For this review, use the dimensioned drawing (mm, ordinates from the lowest corner) and the shaded views. A direction names the side the tool comes from. Coordinates: 2 decimals unless noted, no trailing zeros. Order: outer loops, then holes, each group sorted by start corner. A loop starts at its lowest first (then second) coordinate and runs counter-clockwise, first axis right, second up. Notation, with made-up numbers: M 74,75.5 L 101,75.5 A16 ccw 101,94.5 Z; hole C 17.25,-22 d3. An arc over 180 degrees is marked long. Answer in a Markdown table with one row per item.
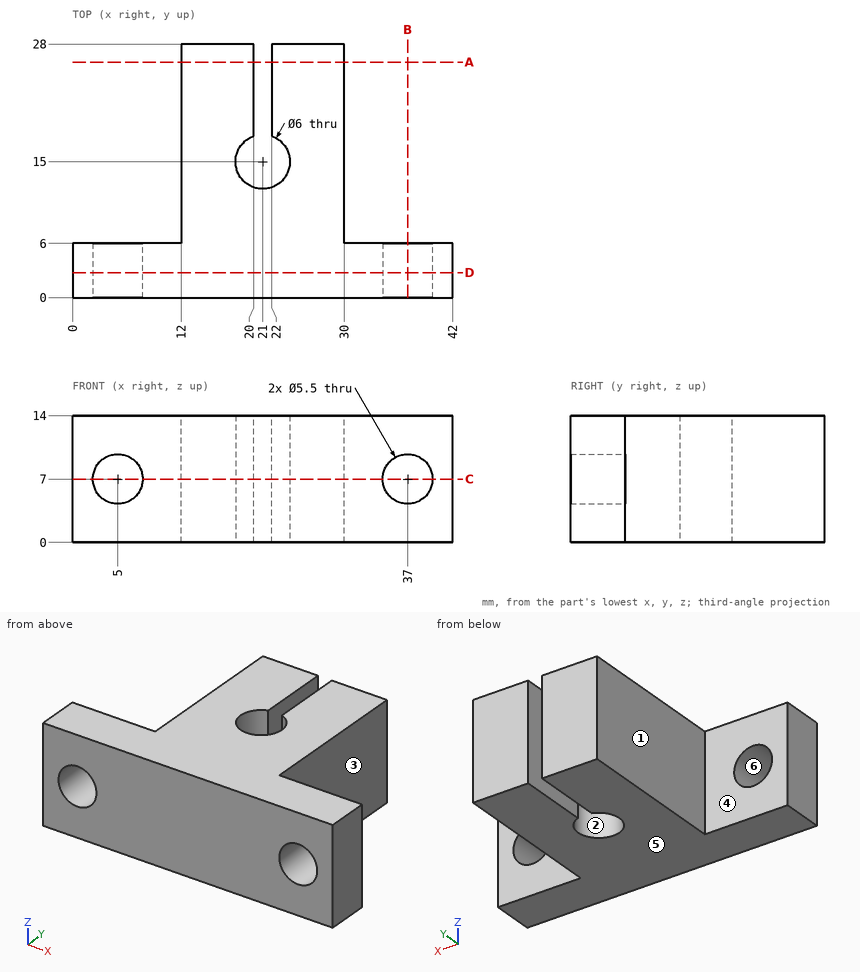
(1) To check wall thickness, follow line 1 (Z direction, x = 37, y = 3.7); line 2 (X direction, y = 21.25, z = 13); line 3 (Y direction, x = 21, z = 10.75). State the ranges of each line that lie inside material, in increasing order. Write a range as [from, to].
Report:
| item | result |
|---|---|
| line 1 | [0, 4.25], [9.75, 14] |
| line 2 | [12, 20], [22, 30] |
| line 3 | [0, 12] |
(2) Take a section at C-C (z = 7). Write out the cut boundary in (x, y), then the cut area to 3 significant figures.
Report:
| item | result |
|---|---|
| outline | M 0,0 L 2.25,0 L 2.25,6 L 0,6 Z; M 7.75,0 L 34.25,0 L 34.25,6 L 30,6 L 30,28 L 22,28 L 22,17.83 A3 cw long 20,17.83 L 20,28 L 12,28 L 12,6 L 7.75,6 Z; M 39.75,0 L 42,0 L 42,6 L 39.75,6 Z |
| area | 534 mm^2 |
(3) Take a section at B-B (x = 37). Write out the cut boundary in (y, z), then the cut area to 3 significant figures.
Report:
| item | result |
|---|---|
| outline | M 0,0 L 6,0 L 6,4.25 L 0,4.25 Z; M 0,9.75 L 6,9.75 L 6,14 L 0,14 Z |
| area | 51.0 mm^2 |
(4) Insertion check: P1, Ø5, axis at y = 24, z = 9.5, coming from the +X side; P2, Ø3.5, axis at x = 5.5, z = 6, coming from the +Y side; P3, Ø7, axis at y = 12, z = 5, coming from the -X side. Each pin has a flat end and moves straight along its axis. Give the tip position at first contact, or say it passes through.
Report:
| item | result |
|---|---|
| P1 | x = 30 |
| P2 | y = 6 |
| P3 | x = 12 |
(5) Take a section at A-A (y = 26). Write out the cut boundary in (x, z), then the cut area to 3 significant figures.
Report:
| item | result |
|---|---|
| outline | M 12,0 L 20,0 L 20,14 L 12,14 Z; M 22,0 L 30,0 L 30,14 L 22,14 Z |
| area | 224 mm^2 |
(6) The part is to be moulded in two halves that separate along Z. For the marked faces 4, 5 and 6, say which applies: +Z half, -Z half, draft (parallel to the pull), parting line (faces both ways), or undercut.
Report:
| item | result |
|---|---|
| face 4 | draft |
| face 5 | -Z half |
| face 6 | undercut |
(7) Take a section at D-D (y = 2.75). Write out the cut boundary in (x, z).
Report:
| item | result |
|---|---|
| outline | M 0,0 L 42,0 L 42,14 L 0,14 Z; hole C 5,7 d5.5; hole C 37,7 d5.5 |
(8) Machinability: for the marked faces 1, 2 and 3, which of the approach directions +Z, -Z, +X, -X, +Y, -Y give a long, thin tool a straight path to every point of the face, cutting with its end or side? Answer none if there is none.
Report:
| item | result |
|---|---|
| face 1 | +Z, -Z, -X, +Y |
| face 2 | +Z, -Z |
| face 3 | +Z, -Z, +X, +Y |
